Part print with two shaded views. Sizes in mm from the minimum x, y, z corner. Round coordinates to 2 decimals unless told otherwise and drop trailing zeros. Order: outer loops, then holes, each group sorted by start corner. A loop starts at its lowest first (then second) coordinate and runs counter-clockwise, first axis right, second up. Notation, with made-up numbers: (-0.75, -28.75) -> (35.25, -28.75) arc R17 ccw to (35.25, -10.75) -> close; hole circle Ø8 at (65, 77). An arc over 180 degrees is marked (long way). Use a Markdown table: item, result. Add a question column.
Item 1: Pin check, flat tips, straight feed: pin 1 (2 mm diameter, centred on x = 198, y = 2.5, fed in from +Z); pin 2 (2 mm diameter, centred on y = 2, z = 64, fed in from -X); pin 3 (6 mm diameter, centred on x = 104.5, z = 143, fed in from -Y); pin 4 (1.5 mm diameter, centred on y = 2, z = 24, fed in from +X). Stop position of each tip, or through.
Item 2: Slice it at C-C, the plane z = 139. Give the cut face in (x, y).
Item 3: Slice it at A-A, the plane x = 15. Give the cut face in (y, z), plus the area to 3 significant figures.
Item 4: Slice it at B-B, the plane y = 1.1. Give the cut face in (x, z).
Item 5: Slice it at D-D, the plane z = 51. Give the cut face in (x, y), plus the area to 3 significant figures.
Item 6: Probe L1, parallel to Z at x = 181.5, y = 3.7; L2, parallel to X at y = 0.7, z = 55; L3, parallel to X at y = 0.7, z = 136.5. List the from-to ranges inside material, lowest first.
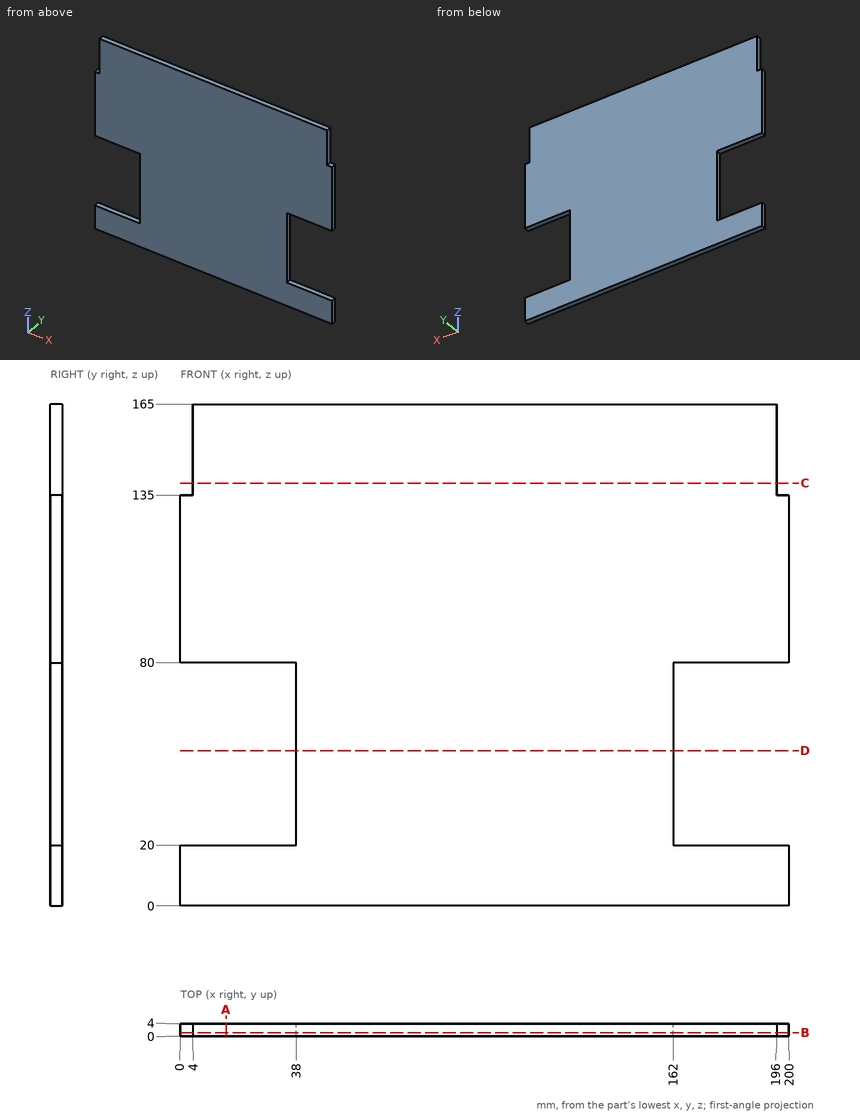
Check sheet entries:
| question | item | result |
|---|---|---|
| 1 | pin 1 | z = 135 |
| 1 | pin 2 | x = 38 |
| 1 | pin 3 | y = 0 |
| 1 | pin 4 | x = 162 |
| 2 | outline | (4, 0) -> (196, 0) -> (196, 4) -> (4, 4) -> close |
| 3 | outline | (0, 0) -> (4, 0) -> (4, 20) -> (0, 20) -> close; (0, 80) -> (4, 80) -> (4, 165) -> (0, 165) -> close |
| 3 | area | 420 mm2 |
| 4 | outline | (0, 0) -> (200, 0) -> (200, 20) -> (162, 20) -> (162, 80) -> (200, 80) -> (200, 135) -> (196, 135) -> (196, 165) -> (4, 165) -> (4, 135) -> (0, 135) -> (0, 80) -> (38, 80) -> (38, 20) -> (0, 20) -> close |
| 5 | outline | (38, 0) -> (162, 0) -> (162, 4) -> (38, 4) -> close |
| 5 | area | 496 mm2 |
| 6 | L1 | 0 to 20, 80 to 165 |
| 6 | L2 | 38 to 162 |
| 6 | L3 | 4 to 196 |
